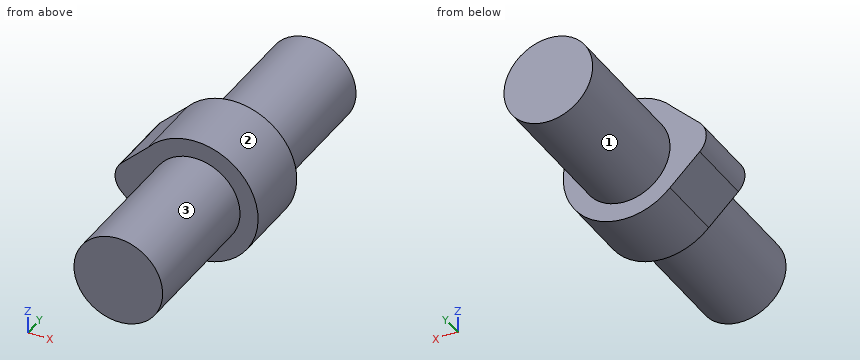
from build123d import *

# Parameters (mm, degrees)
SCHIZZO1_R                   = 6.25
ESTRUSIONE_ESTRUSIONE1_DEPTH = 20
ESTRUSIONE_ESTRUSIONE2_DEPTH = 10
RACCORDO1_R                  = 3
SCHIZZO3_R                   = 6.25
ESTRUSIONE_ESTRUSIONE3_DEPTH = 20


with BuildPart() as part:
    # Schizzo1 → Estrusione-Estrusione1 (new body)
    with BuildSketch(Plane(origin=(0, 0, 0), x_dir=(1, 0, 0), z_dir=(0, 1, 0))):
        with Locations(Location((0, 0, 0), (0, 0, 270))):
            Circle(SCHIZZO1_R)
    extrude(amount=ESTRUSIONE_ESTRUSIONE1_DEPTH)

    # Schizzo2 → Estrusione-Estrusione2 (add)
    with BuildSketch(Plane(origin=(0, 20, 0), x_dir=(1, 0, 0), z_dir=(0, 1, 0))):
        with BuildLine():
            Line((-6.25, 6.194957627), (-12.7, 0))
            Line((-12.7, 0), (-6.657351546, -5.754969192))
            ThreePointArc((-6.657351546, -5.754969192), (8.794891627, -0.299802062), (-6.25, 6.194957627))
        make_face()
    extrude(amount=ESTRUSIONE_ESTRUSIONE2_DEPTH)

    # Raccordo1
    raccordo1_edges = [part.edges().sort_by_distance(p)[0] for p in [
        (-12.7, 25, 0),
    ]]
    fillet(raccordo1_edges, radius=RACCORDO1_R)

    # Schizzo3 → Estrusione-Estrusione3 (add)
    with BuildSketch(Plane(origin=(0, 30, 0), x_dir=(1, 0, 0), z_dir=(0, 1, 0))):
        with Locations(Location((0, 0, 0), (0, 0, 270))):
            Circle(SCHIZZO3_R)
    extrude(amount=ESTRUSIONE_ESTRUSIONE3_DEPTH)


solid = part.part
Source: CAD feature listing. Evaluate the final solid. Frame: model axes, mm. Face numbers are marked on the shaded views. A direction names the side the tool comes from. Give positions to 0.01 mm unless a question says otherwise; leave off trailing zeros. Write each loop counter-clockwise with the first axis right and the second up, starting at its lowest first coordinate (ties: lowest second). Pieces come first, ordered by that corner, then holes. Notation, with made-up numbers: M -26.5,57.5 L 20.5,57.5 A4 ccw 20.5,62.5 Z; hole C 20.5,49.5 d3. An arc over 180 degrees is marked long. Answer as a JSON object with one key per item and string values.
Q1. Cut plane B-B, the plane z = -4.25. Return the cut outline in (x, y), then the cut area to 3 significant figures.
Geometry check:
{"outline": "M -8.28,20 L -4.58,20 L -4.58,0 L 4.58,0 L 4.58,20 L 7.71,20 L 7.71,30 L 4.58,30 L 4.58,50 L -4.58,50 L -4.58,30 L -8.28,30 Z", "area": "526 mm^2"}
Q2. Cut plane C-C, the plane y = 45.5. Return the cut outline in (x, z).
Geometry check:
{"outline": "C 0,0 d12.5"}
Q3. Ray query, line 1 along Y through (x, z) = (3.75, -7); line 2 along Z through (x, y) = (-4, 7.5); line 3 along X through (y, z) = (39.5, -2.75). Return the intervals inside material, ascending.
Geometry check:
{"line 1": "y = 20 to 30", "line 2": "z = -4.8 to 4.8", "line 3": "x = -5.61 to 5.61"}
Q4. Contact query for flat-ended pins moving along their axis: P1, Ø1.5, axis at x = -0.5, y = 16.5, coming from the -Z side; P2, Ø3, axis at x = 5.5, y = 17, coming from the -Z side; P3, Ø8, axis at y = 16.5, z = -3, coming from the -X side. Output: stop coordinate, or through.
Geometry check:
{"P1": "stops at z = -6.25", "P2": "stops at z = -4.8", "P3": "stops at x = -11.17"}
Q5. Cut plane A-A, the plane x = 0. Return the cut outline in (y, z), then the cut area to 3 significant figures.
Geometry check:
{"outline": "M 0,-6.25 L 20,-6.25 L 20,-8.8 L 30,-8.8 L 30,-6.25 L 50,-6.25 L 50,6.25 L 30,6.25 L 30,8.8 L 20,8.8 L 20,6.25 L 0,6.25 Z", "area": "676 mm^2"}
Q6. Cut plane D-D, the plane y = 26. Return the cut outline in (x, z).
Geometry check:
{"outline": "M -10.44,-2.17 L -6.25,-6.19 A8.8 ccw long -6.66,5.75 L -10.43,2.16 A3 ccw Z"}
Q7. Access query for the marked faces 1, 2 and 3. Directions: +Z, -Z, +X, -X, +Y, -Y. A direction counts if a zero-diameter tool reaches every point of the face in a straight line with its end or side. Return the directions, or none.
Geometry check:
{"face 1": "+Y", "face 2": "+Y, -Y", "face 3": "-Y"}
